from build123d import *

# Parameters (mm, degrees)
F0_W     = 120
F0_H     = 40
F0_R     = 4
F1_DEPTH = 200


with BuildPart() as f1:
    # F0 (on Front) → F1 (new body)
    with BuildSketch(Plane.XZ):
        Rectangle(F0_W, F0_H)
        with Locations((50, -10)):
            Circle(F0_R, mode=Mode.SUBTRACT)
        with Locations((-50, 10)):
            Circle(F0_R, mode=Mode.SUBTRACT)
        with Locations((-38, 10)):
            Circle(F0_R, mode=Mode.SUBTRACT)
        with BuildLine():
            ThreePointArc((2.5, 13.122499), (6.732051, 13.605551), (9, 10))
            ThreePointArc((9, 10), (6.732051, 6.394449), (2.5, 6.877501))
            ThreePointArc((2.5, 6.877501), (0, 6), (-2.5, 6.877501))
            ThreePointArc((-2.5, 6.877501), (-9, 10), (-2.5, 13.122499))
            ThreePointArc((-2.5, 13.122499), (0, 14), (2.5, 13.122499))
        make_face(mode=Mode.SUBTRACT)
        with Locations((38, 10)):
            Circle(F0_R, mode=Mode.SUBTRACT)
        with Locations((50, 10)):
            Circle(F0_R, mode=Mode.SUBTRACT)
    extrude(amount=F1_DEPTH)


solid = f1.part
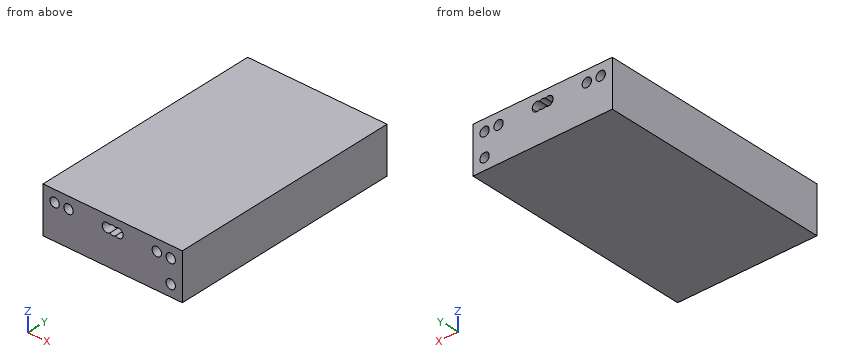
Geometry check sheet. Reference: the model listing, model coordinates, mm. Round coordinates to 2 decimals unless told otherwise and drop trailing zeros. Loops run counter-clockwise (first coordinate to the right, second up) from the corner with the lowest first, then second, coordinate; pieces in that order, holes last.
Item 1: Cross-section at C-C on x = -5. Record the boundary of the cut face in (y, z), then the cut area to 3 significant figures.
Item 2: Thickness scan on line 1 (Z direction, x = 50, y = -87.5); line 2 (Z direction, x = -37.5, y = -130); line 3 (Z direction, x = 52.5, y = -170.5). Record the ranges inside material, lowest first.
Item 3: Cross-section at B-B on y = -115.5. Record the boundary of the cut face in (x, z).
Item 4: Cross-section at A-A on z = -10. Record the boundary of the cut face in (x, y).
Answer sheet:
1. outline: (-200, -20) - (0, -20) - (0, 6) - (-200, 6) - close; (-200, 14) - (0, 14) - (0, 20) - (-200, 20) - close
1. area: 6,400 mm2
2. line 1: z = -20 to -14, -6 to 6, 14 to 20
2. line 2: z = -20 to 6.03, 13.97 to 20
2. line 3: z = -20 to -13.12, -6.88 to 6.88, 13.12 to 20
3. outline: (-60, -20) - (60, -20) - (60, 20) - (-60, 20) - close; hole circle Ø8 at (-50, 10); hole circle Ø8 at (-38, 10); hole (-2.5, 6.88) arc R4 ccw to (2.5, 6.88) arc R4 ccw (long way) to (2.5, 13.12) arc R4 ccw to (-2.5, 13.12) arc R4 ccw (long way) to start; hole circle Ø8 at (38, 10); hole circle Ø8 at (50, -10); hole circle Ø8 at (50, 10)
4. outline: (-60, -200) - (46, -200) - (46, 0) - (-60, 0) - close; (54, -200) - (60, -200) - (60, 0) - (54, 0) - close
